```python
from build123d import *


with BuildPart() as f2:
    # F2: sweep along a path in F1
    with BuildLine(Plane.XZ) as f2_path:
        Line((0, 0), (0, 48.9583745875))
        ThreePointArc((0, 48.9583745875), (-1.2250356126, 53.7542061108), (-4.6, 57.3750247525))
        ThreePointArc((-4.6, 57.3750247525), (3.5, 85), (11.6, 57.3750247525))
        ThreePointArc((11.6, 57.3750247525), (8.2250356126, 53.7542061108), (7, 48.9583745875))
        Line((7, 48.9583745875), (7, -30))
    # F0 (on Top) → F2 (sweep)
    with BuildSketch(Plane.XY):
        with BuildLine():
            Line((0, -4.5), (0, 4.5))
            ThreePointArc((0, 4.5), (-7.1794494718, 0), (0, -4.5))
        make_face()
    sweep(path=f2_path.line)


solid = f2.part
```
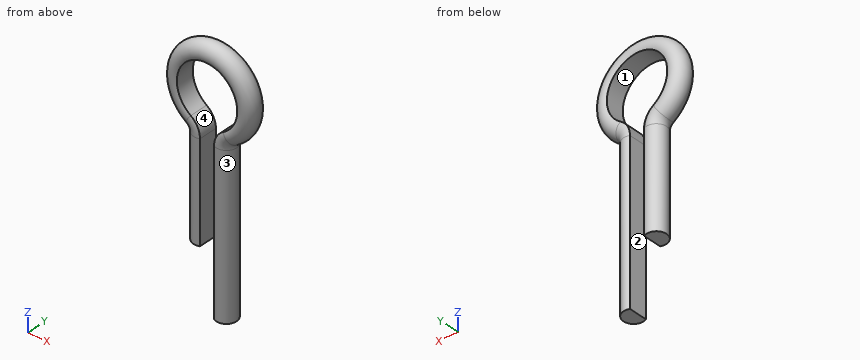
Geometry check sheet. Reference: the model listing, model coordinates, mm. Face numbers are marked on the shaded views. A direction names the side the tool comes from. Round coordinates to 2 decimals unless told otherwise and drop trailing zeros. Loops run counter-clockwise (first coordinate to the right, second up) from the corner with the lowest first, then second, coordinate; pieces in that order, holes last. Notation, with made-up numbers: M 33,6 L 41,6 A23 cw 41,43 Z; hole C 79,33 d6. An arc over 180 degrees is marked long. Return JSON: item names as keys, results as strings. Group by question number.
(1) Set-up check for the marked faces 3 and 4: record each of +Z, -Z, +X, -X, +Y, -Y from which the full face is reachable in a straight line by a thin tool's end or side.
(2) Section check A-A, the plane y = 0. Enter the section's corners in (x, z), and give its area (3 significant figures).
(3) Section check D-D, the plane z = -18. Enter the section's corners in (x, y), and give its area (3 significant figures).
(4) Section check B-B, the plane z = 28. Enter the section's corners in (x, y).
(5) Mould release check, pull along Z, two halves, no side actions. Record for the marked faces 1 and 2: pulls with the +Z half, pulls with the -Z half, needs draft (parallel to the pull), parting line crosses it, or undercut.
(6) Section check C-C, the plane x = 3.5. Enter the section's corners in (y, z), and give its area (3 significant figures).
(7) Go/stop test with flat-tipped pins: pin 1 (4.5 mm diameter, centred on y = 0, z = -7.5, fed in from -X); pin 2 (2.5 mm diameter, centred on y = 1.5, z = 36.5, fed in from +X); pin 3 (2 mm diameter, centred on y = -4, z = 16, fed in from +X). Record where each tip stops, or that it passes through.
(8) Scan lines: line 1 along X through (y, z) = (0, 70); line 2 along X through (y, z) = (1.75, 5); line 3 along Z through (x, y) = (3.5, -0.5). Record each from-to range of solid material in increasing order. Write a range as [from, to].
Data:
{
 "1": {"face 3": "-Z", "face 4": "+Y, -Y"},
 "2": {"outline": "M -8.48,51.33 A2.82 cw -7.18,48.96 L -7.18,0 L 0,0 L 0,48.96 A10 ccw -4.6,57.38 A15 cw long 11.6,57.38 A10 ccw 7,48.96 L 7,-30 L 14.18,-30 L 14.18,48.96 A2.82 cw 15.48,51.33 A22.18 ccw long Z", "area": "1,700 mm²"},
 "3": {"outline": "M 7,-4.5 A5 ccw long 7,4.5 Z", "area": "60.4 mm²"},
 "4": {"outline": "M 0,-4.5 L 0,4.5 A5 ccw long Z; M 7,-4.5 A5 ccw long 7,4.5 Z"},
 "5": {"face 1": "undercut", "face 2": "needs draft"},
 "6": {"outline": "M -4.5,85 L 4.5,85 A5 ccw long Z", "area": "60.4 mm²"},
 "7": {"pin 1": "x = 7", "pin 2": "x = 14.17", "pin 3": "x = 13.18"},
 "8": {"line 1": "[-18.68, -11.5], [18.5, 25.68]", "line 2": "[-6.86, 0], [7, 13.86]", "line 3": "[85, 92.15]"}
}
